The drawing under review shows one solid part. Ordinate dimensions are in mm from its lowest x, y, z. A direction names the side the tool comes from. Round coordinates to 2 decimals unless told otherwise and drop trailing zeros. Write each loop counter-clockwise with the first axis right and the second up, starting at its lowest first coordinate (ties: lowest second). Pieces come first, ordered by that corner, then holes. Notation, with made-up numbers: (84.25, 1.25) -> (138.25, 1.25) arc R20 cw to (138.25, 33.25) -> close; hole circle Ø1 at (10, 86). An arc over 180 degrees is marked (long way). Write item = value, one per line. Start each with the question number.
Item 1: Machinability: for the marked faces 1 and 2, which of the approach directions +Z, -Z, +X, -X, +Y, -Y give a long, thin tool a straight path to every point of the face, cutting with its end or side? Answer none if there is none.
Item 2: For pin 1 Ø11.5 at (y, z) = (41, 89) entering from +X; pin 2 Ø2 at (x, z) = (20, 103) entering from +Y, all flat-tipped, find the tip position at first contact; note any pin that passes through.
Item 3: Add section B-B, the plane y = 33. State the section outline as (x, z) points, then the cut area to 3 significant figures.
Item 4: To check wall thickness, follow L1, parallel to X at y = 29, z = 136.5; L2, parallel to Y at x = 10, z = 129. State the ranges of each line that lie inside material, in increasing order.
Item 5: Add section A-A, the plane z = 22.5. State the section outline as (x, y) points, then the cut area to 3 significant figures.
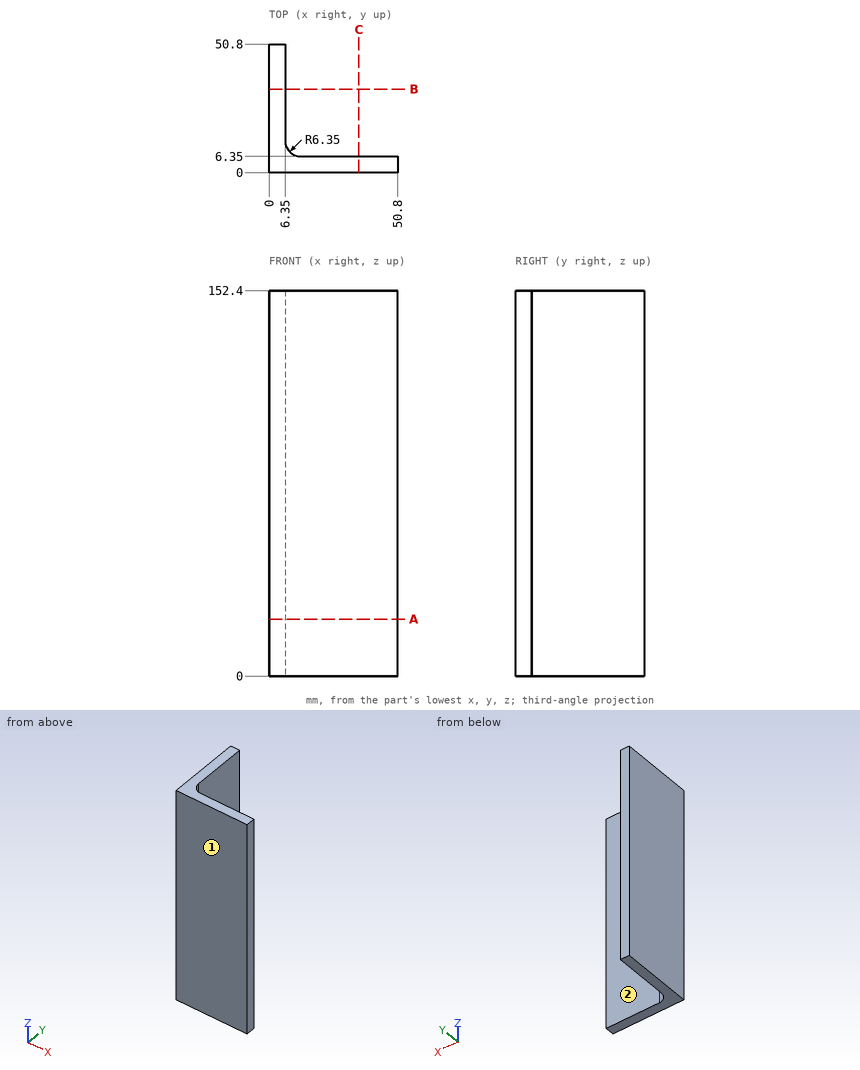
Result set:
q1.face_1 = +Z, -Z, +X, -X, -Y
q1.face_2 = +Z, -Z, +X, +Y
q2.pin_1 = 6.35
q2.pin_2 = 6.35
q3.outline = (0, 0) -> (6.35, 0) -> (6.35, 152.4) -> (0, 152.4) -> close
q3.area = 968 mm²
q4.L1 = 0 to 6.35
q4.L2 = 0 to 6.95
q5.outline = (0, 0) -> (50.8, 0) -> (50.8, 6.35) -> (12.7, 6.35) arc R6.35 cw to (6.35, 12.7) -> (6.35, 50.8) -> (0, 50.8) -> close
q5.area = 613 mm²
